from build123d import *

# Parameters (mm, degrees)
F1_DEPTH = 63.5
F0_W     = 25.4
F0_H     = 19.05
F2_DEPTH = 50.8
F3_DEPTH = 15.875


with BuildPart() as f1:
    # F0 (on Front) → F1 (new body, symmetric)
    with BuildSketch(Plane.XZ):
        Polygon((22.225, 9.525), (-41.275, 9.525), (-41.275, -9.525), (41.275, -9.525), (41.275, 9.525), align=None)
    extrude(amount=F1_DEPTH, both=True)

    # F0 (on Front) → F2 (join)
    with BuildSketch(Plane.XZ):
        with BuildLine():
            Line((22.225, 27.0002), (22.225, 9.525))
            Line((22.225, 9.525), (41.275, 9.525))
            Line((41.275, 9.525), (41.275, 27.0002))
            ThreePointArc((41.275, 27.0002), (45.9246798487, 38.2255201513), (57.15, 42.8752))
            Line((57.15, 42.8752), (60.325, 42.8752))
            Line((60.325, 42.8752), (60.325, 61.9252))
            Line((60.325, 61.9252), (57.15, 61.9252))
            add(Edge.make_bspline(
                [(55.1300589584, 61.8667378721), (55.8023663575, 61.8895709861), (56.4757096001, 61.9090664162), (57.15, 61.9252)],
                knots=[110.0549330029, 110.0549330029, 110.0549330029, 110.0549330029, 111.5045361635, 111.5045361635, 111.5045361635, 111.5045361635], degree=3))
            ThreePointArc((55.1300589584, 61.8667378721), (31.7501765176, 50.9711113732), (22.225, 27.0002))
        make_face()
        with Locations((73.025, 52.4002)):
            Rectangle(F0_W, F0_H)
    extrude(amount=F2_DEPTH)

    # F0 (on Front) → F3 (join)
    with BuildSketch(Plane.XZ):
        with BuildLine():
            add(Edge.make_bspline(
                [(-41.275, 9.525), (-40.983522632, 39.1614563613), (4.0879891143, 60.1332311464), (55.1300589584, 61.8667378721)],
                knots=[0, 0, 0, 0, 110.0549330029, 110.0549330029, 110.0549330029, 110.0549330029], degree=3))
            Line((-41.275, 9.525), (22.225, 9.525))
            Line((22.225, 9.525), (22.225, 27.0002))
            ThreePointArc((22.225, 27.0002), (31.7501765176, 50.9711113732), (55.1300589584, 61.8667378721))
        make_face()
    extrude(amount=F3_DEPTH)


solid = f1.part
CAD build for the part. Positions are in the model's coordinates, mm. A direction names the side the tool comes from. Round coordinates to 2 decimals unless told otherwise and drop trailing zeros. Write each loop counter-clockwise with the first axis right and the second up, starting at its lowest first coordinate (ties: lowest second). Pieces come first, ordered by that corner, then holes. Notation, with made-up numbers: M 83,80 L 103,80 A23 cw 103,102 Z; hole C 65.5,-35 d10. An arc over 180 degrees is marked long. Use a Markdown table: item, result. Add a question column.
1. Slice it at A-A on y = 43.5. Give the cut face in (x, z) (3 decimals).
2. Flat gauge pins, fed straight in: P1, Ø1, axis at x = 31.5, z = 14, coming from the -Y side; P2, Ø19, axis at x = 9, y = 20.5, coming from the +Z side (3 decimals); P3, Ø12, axis at x = 31, z = 21.5, coming from the +Y side. Where does each tip first touch, or does it go through?
3. Slice it at B-B on z = 5.5. Give the cut face in (x, y) (3 decimals), then the cut area to 3 significant figures.
4. Drill centre lines: probe 1 along Y at (x, z) = (-5.5, 27) (3 decimals); probe 2 along X at (y, z) = (-4.5, 0) (3 decimals); probe 3 along Z at (x, y) = (68, -23). Where is each one in solid material? Low to high.
5. 3-axis set-ups, long thin cutter, end or side, ignore diameter. For faces 1 (the face through (46, -50.8, 42)), 2 (the face through (23, 0, 36)), 3 (the face through (41.275, -1, 4)): which of +Z, -Z, +X, -X, +Y, -Y reach the whole face in a straight line?
Reply:
| question | item | result |
|---|---|---|
| 1 | outline | M -41.275,-9.525 L 41.275,-9.525 L 41.275,9.525 L -41.275,9.525 Z |
| 2 | P1 | stops at y = -50.8 |
| 2 | P2 | stops at z = 9.525 |
| 2 | P3 | stops at y = 0 |
| 3 | outline | M -41.275,-63.5 L 41.275,-63.5 L 41.275,63.5 L -41.275,63.5 Z |
| 3 | area | 10,500 mm^2 |
| 4 | probe 1 | y = -15.875 to 0 |
| 4 | probe 2 | x = -41.275 to 41.275 |
| 4 | probe 3 | z = 42.88 to 61.93 |
| 5 | face 1 | +Z, +X, -X, -Y |
| 5 | face 2 | +Z, +X, -X, +Y |
| 5 | face 3 | -Z, +X, +Y, -Y |
